Check sheet for the modelled part. Datum: model origin and axes. Units: mm. A direction names the side the tool comes from. Round coordinates to 2 decimals unless told otherwise and drop trailing zeros. Write each loop counter-clockwise with the first axis right and the second up, starting at its lowest first coordinate (ties: lowest second). Pieces come first, ordered by that corner, then holes.
Item 1: Cross-section at C-C on y = 2.75. Enter the section's corners in (x, z).
Item 2: Material ranges on line 1 (Y direction, x = 5.75, z = -2); line 2 (X direction, y = -0.5, z = 6); line 3 (Z direction, x = 1, y = -0.25), recorded low to high.
Item 3: Cross-section at A-A on z = -0.5. Enter the section's corners in (x, y).
Item 4: Tool access check on faces 1 (the flat face through (8, -3.238, 0)), 2 (the flat face through (7, 1, 11.646)), 3 (the flat face through (8, 1, -11.646)), 4 (the flat face through (7.554, -3.095, -10.669)). Record the directions out of +Z, -Z, +X, -X, +Y, -Y that give a thin tool (end or side, any length) a straight path to the whole face; none if there is none.
Item 5: Cross-section at B-B on x = 4.25. Enter the section's corners in (y, z).
Item 6: Cross-section at D-D on x = -2. Enter the section's corners in (y, z), plus the area to 3 significant figures.
Item 7: Release check for a two-part mould opening along Y. For faces 5 (the flat face through (7.554, -2.426, 9.905)), 6 (the flat face through (1.854, 3.5, -1.1)), 7 (the flat face through (0, -4.254, 0)) record: +Y half, -Y half, draft (parallel to the pull), parting line (faces both ways), or undercut.
Item 8: Go/stop test with flat-tipped pins: pin 1 Ø3 at (x, y) = (8, 2.5) entering from +Z; pin 2 Ø2.5 at (x, y) = (8.5, 1.5) entering from -Z; pin 3 Ø3 at (y, z) = (0, 6) entering from +X. Record where each tip stops, or that it passes through.
Autodesk Inventor part; units mm, degrees
ref_plane "YZ Plane" through (0, 0, 0) normal (1, 0, 0) x (0, 1, 0)
ref_plane "XZ Plane" through (0, 0, 0) normal (0, 1, 0) x (-1, 0, 0)
ref_plane "XY Plane" through (0, 0, 0) normal (0, 0, 1) x (1, 0, 0)
sketch "Sketch1" plane through (0, 0, 0) normal (0, 1, 0) x (-1, 0, 0)
  line L0 (-11.8618, -11.6459) -> (11.8618, -11.6459)
  line L1 (11.8618, -11.6459) -> (11.8618, 11.6459)
  line L2 (11.8618, 11.6459) -> (-11.8618, 11.6459)
  line L3 (-11.8618, 11.6459) -> (-11.8618, -11.6459)
  line L4 (-11.8618, -11.6459) -> (11.8618, 11.6459) construction
  line L5 (11.8618, -11.6459) -> (-11.8618, 11.6459) construction
  point P0 (0, 0)
  dimension "d0" = 23.2918
  dimension "d1" = 23.7236
extrude "Extrusion1" add sketch "Sketch1" along normal mid plane 8.509
sketch "Sketch2" plane through (0, 4.2545, 0) normal (0, 1, 0) x (1, 0, 0)
  line L0 (-11.8618, 11.6459) -> (-11.8618, -11.6459)
  line L1 (11.8618, 11.6459) -> (-11.8618, 11.6459)
  line L2 (-11.8618, -11.6459) -> (1.8542, -11.6459)
  line L3 (1.8542, -11.6459) -> (1.8542, 11.6459)
  line L4 (1.8542, 11.6459) -> (-11.8618, 11.6459)
  line L5 (-11.8618, 11.6459) -> (-11.8618, -11.6459)
  point P0 (0, 0)
  dimension "d4" = 13.716
extrude "Extrusion2" cut sketch "Sketch2" against normal blind 1.0414
sketch "Sketch3" plane through (0, 3.2131, 0) normal (0, 1, 0) x (1, 0, 0)
  line L0 (-11.8618, -11.6459) -> (-11.8618, 11.6459)
  line L1 (1.8542, 11.6459) -> (1.8542, -11.6459)
  line L2 (-11.8618, -10.5791) -> (1.8542, -10.5791)
  line L3 (1.8542, -10.5791) -> (1.8542, 10.5791)
  line L4 (1.8542, 10.5791) -> (-11.8618, 10.5791)
  line L5 (-11.8618, 10.5791) -> (-11.8618, -10.5791)
  line L6 (1.8542, -11.6459) -> (-11.8618, -11.6459)
  line L7 (-11.8618, 11.6459) -> (1.8542, 11.6459)
  line L8 (1.8542, -11.6459) -> (1.8542, -10.5791)
  line L9 (1.8542, 11.6459) -> (1.8542, 10.5791)
  point P0 (0, 0)
  dimension "d7" = 1.0668
  dimension "d8" = 21.1582
  dimension "d9" = 1.0668
extrude "Extrusion3" cut sketch "Sketch3" against normal up to surface (7.4676 mm away) contours L0 L2 L1 L6 | L0 L7 L1 L4
sketch "Sketch4" plane through (1.8542, 4.2545, -11.6459) normal (-1, 0, 0) x (0, 0, 1)
  line L0 (-2.0701, 0) -> (25.3619, 0)
  line L1 (25.3619, 0) -> (25.3619, -8.509)
  line L2 (25.3619, -8.509) -> (-2.0701, -8.509)
  line L3 (-2.0701, -8.509) -> (-2.0701, 0)
  line L4 (23.2918, -8.509) -> (22.225, -8.509)
  line L5 (0, 0) -> (23.2918, 0)
  line L6 (23.2918, 0) -> (23.2918, -8.509)
  line L7 (0, -8.509) -> (0, 0)
  point P0 (11.6459, -4.2545)
  dimension "d12" = 27.432
  dimension "d13" = 2.0701
  dimension "d14" = 2.0701
extrude "Extrusion4" add sketch "Sketch4" against normal blind 1.27 contours L0 L7 L2 L3 | L0 L1 L2 L6
sketch "Sketch5" plane through (11.8618, -4.2545, -11.6459) normal (1, 0, 0) x (0, 0, -1)
  line L0 (-23.2918, 8.509) -> (-23.2918, 0)
  line L1 (-23.2918, 2.286) -> (-21.3106, 0)
  line L2 (-21.3106, 0) -> (-1.9812, 0)
  line L3 (0, 0) -> (-23.2918, 0)
  line L4 (0, 0) -> (0, 8.509)
  line L5 (0, 2.286) -> (-1.9812, 0)
  point P0 (-11.6459, 4.2545)
  dimension "d17" = 19.3294
  dimension "d20" = 6.223
  dimension "d21" = 139.086
  dimension "d22" = 139.086
extrude "Extrusion5" cut sketch "Sketch5" against normal up to surface (8.7376 mm away)
sketch "Sketch6" plane through (11.8618, 4.2545, 11.6459) normal (1, 0, 0) x (0, 0, -1)
  line L0 (21.3106, -8.509) -> (23.2918, -6.223)
  line L1 (23.2918, -6.223) -> (23.2918, 0)
  line L2 (0, 0) -> (23.2918, 0)
  line L3 (0, -6.223) -> (0, 0)
  line L4 (0, -6.223) -> (1.9812, -8.509)
  line L5 (21.3106, -8.509) -> (1.9812, -8.509)
  line L6 (2.4451, -7.493) -> (1.016, -5.844)
  line L7 (1.016, -5.844) -> (1.016, -1.016)
  line L8 (1.016, -1.016) -> (22.2758, -1.016)
  line L9 (22.2758, -1.016) -> (22.2758, -5.844)
  line L10 (22.2758, -5.844) -> (20.8467, -7.493)
  line L11 (20.8467, -7.493) -> (2.4451, -7.493)
  point P0 (11.6459, -4.2545)
  dimension "d25" = 1.016
extrude "Extrusion6" cut sketch "Sketch6" against normal up to surface (8.7376 mm away) contours L6 L7 L8 L9 L10 L11
equation "\"d7\" = d9"
equation "\"d13\" = d14"
equation "\"d21\" = d22"
properties part number "MolexConnector"
Response values:
1. outline: (-11.86, -10.58) - (1.85, -10.58) - (1.85, -13.72) - (3.12, -13.72) - (3.12, -11.65) - (11.86, -11.65) - (11.86, -10.63) - (3.12, -10.63) - (3.12, 10.63) - (11.86, 10.63) - (11.86, 11.65) - (3.12, 11.65) - (3.12, 13.72) - (1.85, 13.72) - (1.85, 10.58) - (-11.86, 10.58) - close
2. line 1: y = -4.25 to -3.24, 3.24 to 4.25
2. line 2: x = -11.86 to 3.12
2. line 3: z = -10.58 to 10.58
3. outline: (-11.86, -4.25) - (11.86, -4.25) - (11.86, -3.24) - (3.12, -3.24) - (3.12, 3.24) - (11.86, 3.24) - (11.86, 4.25) - (1.85, 4.25) - (1.85, 3.21) - (-11.86, 3.21) - close
4. face 1: +X
4. face 2: +Z, +X, +Y, -Y
4. face 3: -Z, +X, +Y, -Y
4. face 4: -Z, +X, -Y
5. outline: (-4.25, -9.66) - (-1.97, -11.65) - (4.25, -11.65) - (4.25, 11.65) - (-1.97, 11.65) - (-4.25, 9.66) - close; hole (-3.24, -9.2) - (-1.59, -10.63) - (3.24, -10.63) - (3.24, 10.63) - (-1.59, 10.63) - (-3.24, 9.2) - close
6. outline: (-4.25, -10.58) - (3.21, -10.58) - (3.21, 10.58) - (-4.25, 10.58) - close
6. area: 158 mm2
7. face 5: undercut
7. face 6: draft
7. face 7: -Y half
8. pin 1: stops at z = 11.65
8. pin 2: stops at z = -11.65
8. pin 3: stops at x = 3.12
